Geometry: see drawing. Coordinates: mm, zero at the bounding-box minimum. A direction names the side the tool comes from. Give positions to 0.01 mm unless a question says otherwise; leave off trailing zeros. Write each loop counter-clockwise with the first axis right and the second up, starting at its lowest first coordinate (ties: lowest second). Pieces come first, ordered by that corner, then holes. Notation, with made-up numbers: M 34,26.5 L 42,26.5 A16 cw 42,35.5 Z; hole C -38.75,63 d2. An arc over 180 degrees is marked long. Use CSV: the item, a comma, the result in double quotes. Start each with the question number.
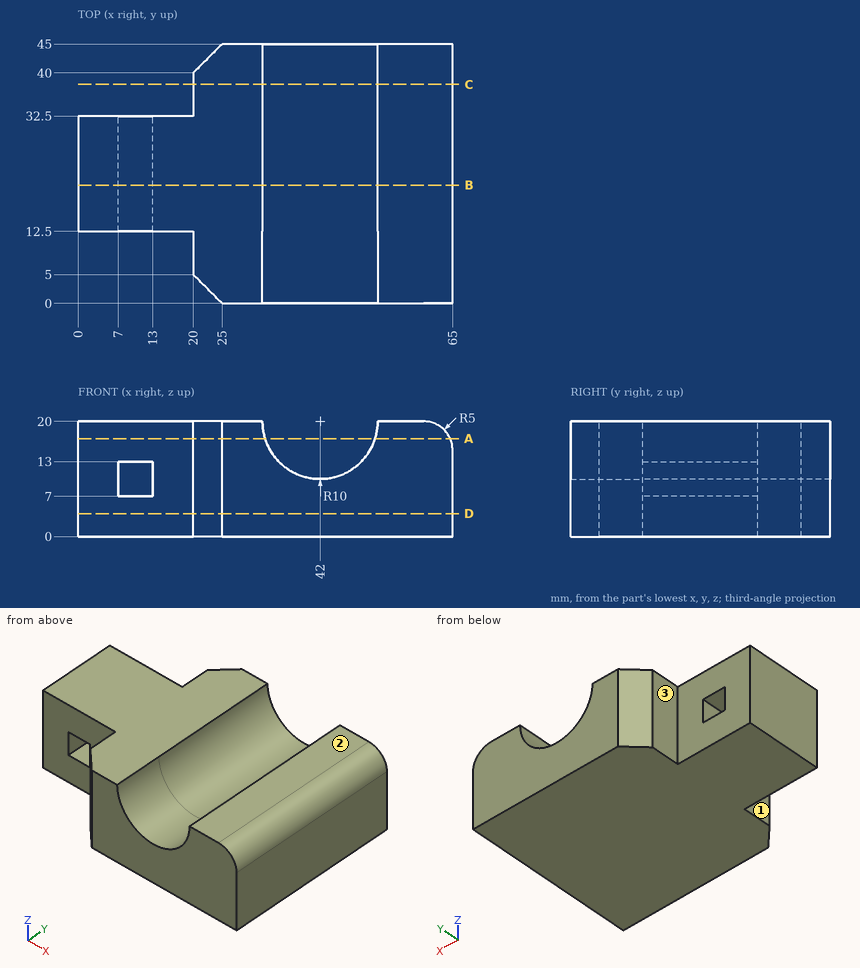
1. Section C-C on y = 38. Return loops of the section in (x, z).
2. Section B-B on y = 20.5. Return loops of the section in (x, z).
3. Access query for the marked faces 1, 2 and 3. Directions: +Z, -Z, +X, -X, +Y, -Y. A direction counts if a zero-diameter tool reaches every point of the face in a straight line with its end or side. Return the directions, or none.
4. Section D-D on z = 4. Return loops of the section in (x, y), then the cut area to 3 significant figures.
5. Line query: probe 1 along Y at (x, z) = (6.5, 15.5); probe 2 along X at (y, z) = (24, 12.5); probe 3 along X at (y, z) = (6, 12.5). Output: solid intervals per line, ascending.
6. First-contact query: pin 1 (8 mm diameter, centred on y = 8, z = 10.5, fed in from -X); pin 2 (12 mm diameter, centred on x = 13.5, z = 16, fed in from -Y); pin 3 (6 mm diameter, centred on x = 19, z = 8.5, fed in from -Y). Flat tips, straight axial feed; report the tip coordinate or a pass-through.
7. Section A-A on z = 17. Return loops of the section in (x, y).
Resolved:
1,outline,"M 20,0 L 65,0 L 65,15 A5 ccw 60,20 L 52,20 A10 cw 32,20 L 20,20 Z"
2,outline,"M 0,0 L 65,0 L 65,15 A5 ccw 60,20 L 52,20 A10 cw 32,20 L 0,20 Z; hole M 7,7 L 13,7 L 13,13 L 7,13 Z"
3,face 1,"+Z, -Z, -X, -Y"
3,face 2,"+Z, +X, -X, +Y, -Y"
3,face 3,"+Z, -Z, -X, +Y"
4,outline,"M 0,12.5 L 20,12.5 L 20,5 L 25,0 L 65,0 L 65,45 L 25,45 L 20,40 L 20,32.5 L 0,32.5 Z"
4,area,"2,400 mm2"
5,probe 1,"y = 12.5 to 32.5"
5,probe 2,"x = 0 to 7, 13 to 35.39, 48.61 to 65"
5,probe 3,"x = 20 to 35.39, 48.61 to 65"
6,pin 1,"stops at x = 20"
6,pin 2,"stops at y = 12.5"
6,pin 3,"stops at y = 3"
7,outline,"M 0,12.5 L 20,12.5 L 20,5 L 25,0 L 32.46,0 L 32.46,45 L 25,45 L 20,40 L 20,32.5 L 0,32.5 Z; M 51.54,0 L 64.58,0 L 64.58,45 L 51.54,45 Z"
